Drawing for the job (mm, zero at the part's lowest x, y, z). A direction names the side the tool comes from. Give positions to 0.01 mm unless a question says otherwise; leave off trailing zeros. Order: outer loops, then holes, each group sorted by start corner. A loop starts at its lowest first (then second) coordinate and runs counter-clockwise, first axis right, second up. Notation, with made-up numbers: M -37,87.25 L -26,87.25 A26 cw -26,123.25 Z; hole C 70,52.5 d9. An arc over 180 degrees is marked long. Answer as a JSON object with one key per item and string values.
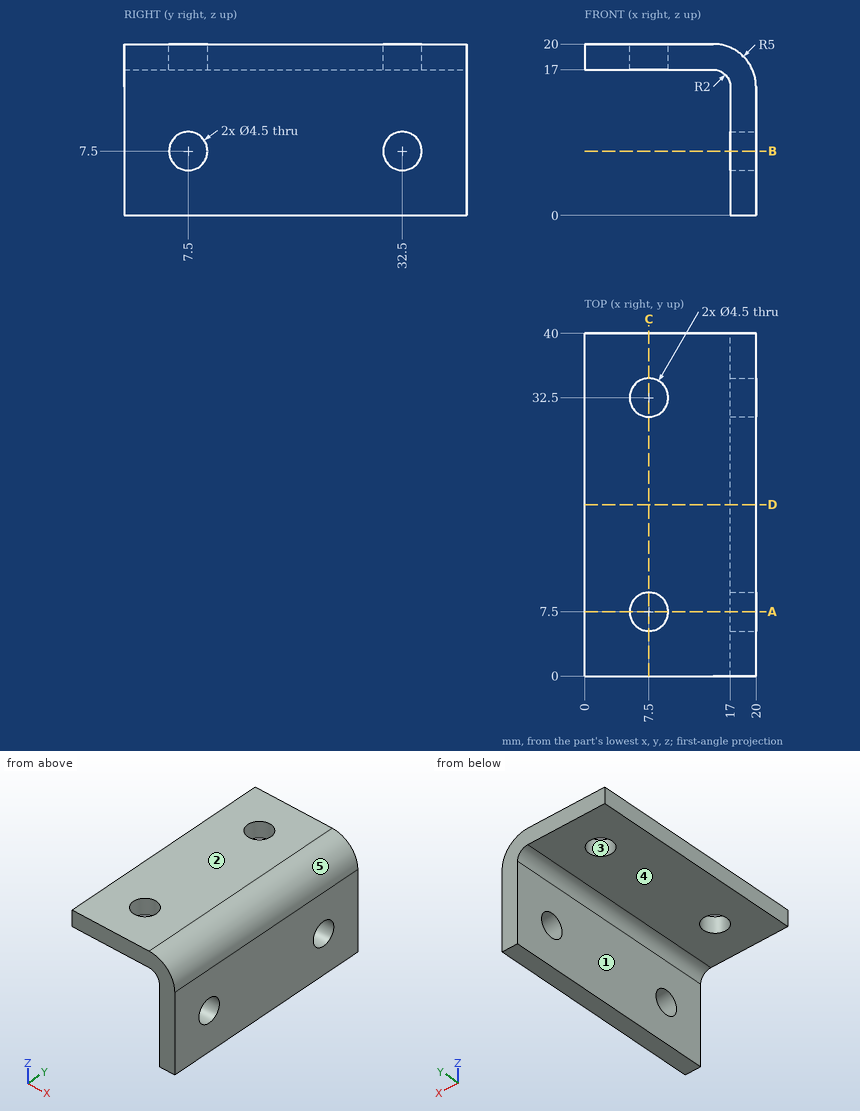
1. Two-plate mould, pull along X, no slides. Class the marked faces 1, 2 and 3: +X half, -X half, draft (parallel to the pull), parting line (faces both ways), or undercut.
Worked answers:
{"face 1": "-X half", "face 2": "draft", "face 3": "undercut"}
2. Cut at D-D on y = 20. Give the cut face in (x, z), plus the area to 3 significant figures.
Worked answers:
{"outline": "M 0,17 L 15,17 A2 cw 17,15 L 17,0 L 20,0 L 20,15 A5 ccw 15,20 L 0,20 Z", "area": "106 mm^2"}
3. Pin check, flat tips, straight feed: P1, Ø6, axis at x = 4.5, y = 17, coming from the -Z side; P2, Ø8, axis at y = 27, z = 7, coming from the -X side. Stop position of each tip, or through.
Worked answers:
{"P1": "stops at z = 17", "P2": "stops at x = 17"}
4. Cut at C-C on x = 7.5. Give the cut face in (y, z), plus the area to 3 significant figures.
Worked answers:
{"outline": "M 0,17 L 5.25,17 L 5.25,20 L 0,20 Z; M 9.75,17 L 30.25,17 L 30.25,20 L 9.75,20 Z; M 34.75,17 L 40,17 L 40,20 L 34.75,20 Z", "area": "93.0 mm^2"}
5. Which spindle directions (+Z, -Z, +X, -X, +Y, -Y) get a long thin tool onto all of the face, cutting with end or side? Do the marked faces 4 and 5. Say none if no direction does.
Worked answers:
{"face 4": "-Z, -X, +Y, -Y", "face 5": "+Z, +X, +Y, -Y"}
6. Probe line 1 along Y through (x, z) = (17.9, 7.5); line 2 along X through (y, z) = (24.5, 8.75). List the from-to ranges inside material, lowest first.
Worked answers:
{"line 1": "y = 0 to 5.25, 9.75 to 30.25, 34.75 to 40", "line 2": "x = 17 to 20"}
7. Cut at B-B on z = 7.5. Give the cut face in (x, y).
Worked answers:
{"outline": "M 17,0 L 20,0 L 20,5.25 L 17,5.25 Z; M 17,9.75 L 20,9.75 L 20,30.25 L 17,30.25 Z; M 17,34.75 L 20,34.75 L 20,40 L 17,40 Z"}
8. Cut at A-A on y = 7.5. Give the cut face in (x, z), plus the area to 3 significant figures.
Worked answers:
{"outline": "M 0,17 L 5.25,17 L 5.25,20 L 0,20 Z; M 9.75,17 L 15,17 A2 cw 17,15 L 17,9.75 L 20,9.75 L 20,15 A5 ccw 15,20 L 9.75,20 Z; M 17,0 L 20,0 L 20,5.25 L 17,5.25 Z", "area": "79.5 mm^2"}
